Geometry check sheet. Reference: drawing and pictorial views, mm from the part's lowest x, y, z. Round coordinates to 2 decimals unless told otherwise and drop trailing zeros. Write each loop counter-clockwise with the first axis right and the second up, starting at its lowest first coordinate (ties: lowest second). Pieces come first, ordered by that corner, then holes.
Item 1: Section check B-B, the plane z = 1.8. Record the cut outline in (x, y), plus the area to 3 significant figures.
Item 2: Depth check by flat-ended pin: pin 1 (3.5 mm diameter, centred on x = 25, y = 3, fed in from +Z). Enter the tip coordinate at first touch or a pass-through.
Item 3: Material ranges on line 1 along X through (y, z) = (17, 0.8); line 2 along Y through (x, z) = (25, 0.4); line 3 along X through (y, z) = (2, 2.25), recorded low to high.
Item 4: Release check for a two-part mould opening along X. For the marked faces 1, 2, 3 and 4 record: pulls with the +X half, pulls with the -X half, needs draft (parallel to the pull), parting line crosses it, or undercut.
Item 5: Section check A-A, the plane z = 0.4. Record the cut outline in (x, y), plus the area to 3 significant figures.
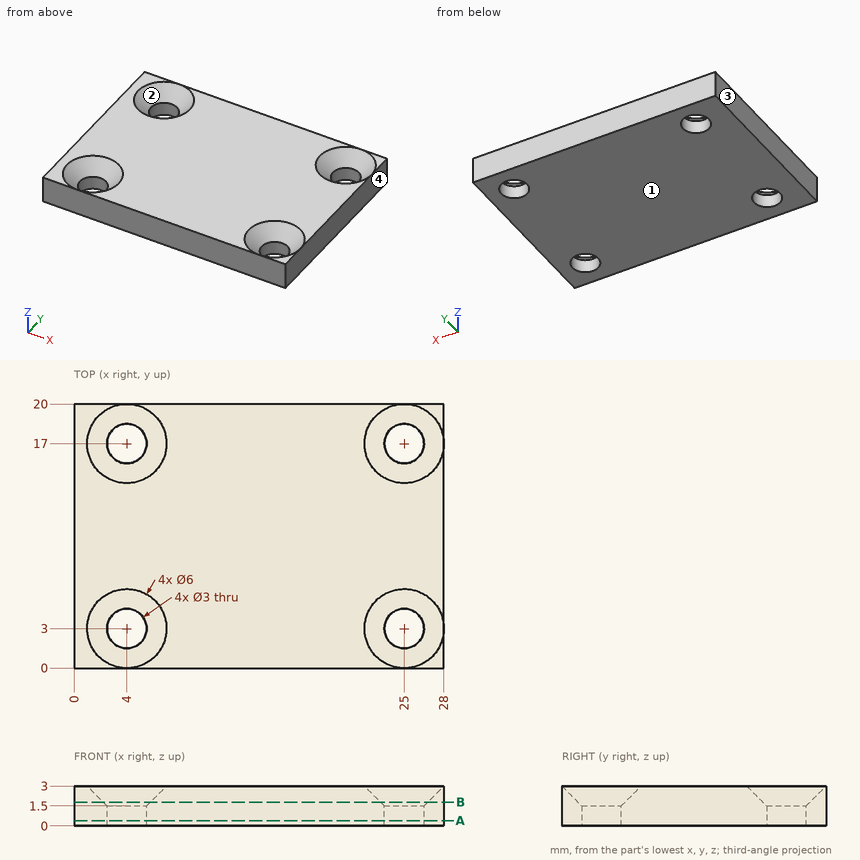
Values found:
1. outline: (0, 0) - (28, 0) - (28, 20) - (0, 20) - close; hole circle Ø3.6 at (4, 3); hole circle Ø3.6 at (4, 17); hole circle Ø3.6 at (25, 3); hole circle Ø3.6 at (25, 17)
1. area: 519 mm2
2. pin 1: stops at z = 1.75
3. line 1: x = 0 to 2.5, 5.5 to 23.5, 26.5 to 28
3. line 2: y = 0 to 1.5, 4.5 to 15.5, 18.5 to 20
3. line 3: x = 0 to 1.98, 6.02 to 22.98, 27.02 to 28
4. face 1: needs draft
4. face 2: undercut
4. face 3: pulls with the -X half
4. face 4: pulls with the +X half
5. outline: (0, 0) - (28, 0) - (28, 20) - (0, 20) - close; hole circle Ø3 at (4, 3); hole circle Ø3 at (4, 17); hole circle Ø3 at (25, 3); hole circle Ø3 at (25, 17)
5. area: 532 mm2
